Source: three-view drawing plus pictorial views. Frame: mm from the lowest corner of the part. Coordinates: 2 decimals unless noted, no trailing zeros. Loops run counter-clockwise (first coordinate to the right, second up) from the corner with the lowest first, then second, coordinate; pieces in that order, holes last. Notation, with made-up numbers: M -26,-40 L 9,-40 A4 ccw 9,-36 Z; hole C -18,-24 d10. An arc over 180 degrees is marked long. Use a Markdown table: item, result. Add a question column.
1. Section B-B on z = 5. Output: boundary loops of the cut face in (x, y).
2. Section D-D on x = 18. Output: boundary loops of the cut face in (y, z), then the cut area to 3 significant figures.
3. Pin query (flat end, axial travel): pin 1 (6 mm diameter, centred on x = 38, y = 9, fed in from +Z); pin 2 (2 mm diameter, centred on y = 3, z = 3.5, fed in from +X); pin 3 (2 mm diameter, centred on y = 20.5, z = 1, fed in from -X); pin 4 (4 mm diameter, centred on x = 79.5, z = 2.5, fed in from -Y). Return the tip coordinate at first contact, or that it passes through.
4. Line query: L1, parallel to Y at x = 12.25, z = 5; L2, parallel to Y at x = 4.5, z = 5; L3, parallel to X at y = 7, z = 9.5. Output: solid intervals per line, ascending. Write a range as [from, to].
5. Section C-C on y = 13. Output: boundary loops of the cut face in (x, z), then the cut area to 3 significant figures.
6. Section A-A on x = 5. Output: boundary loops of the cut face in (y, z).
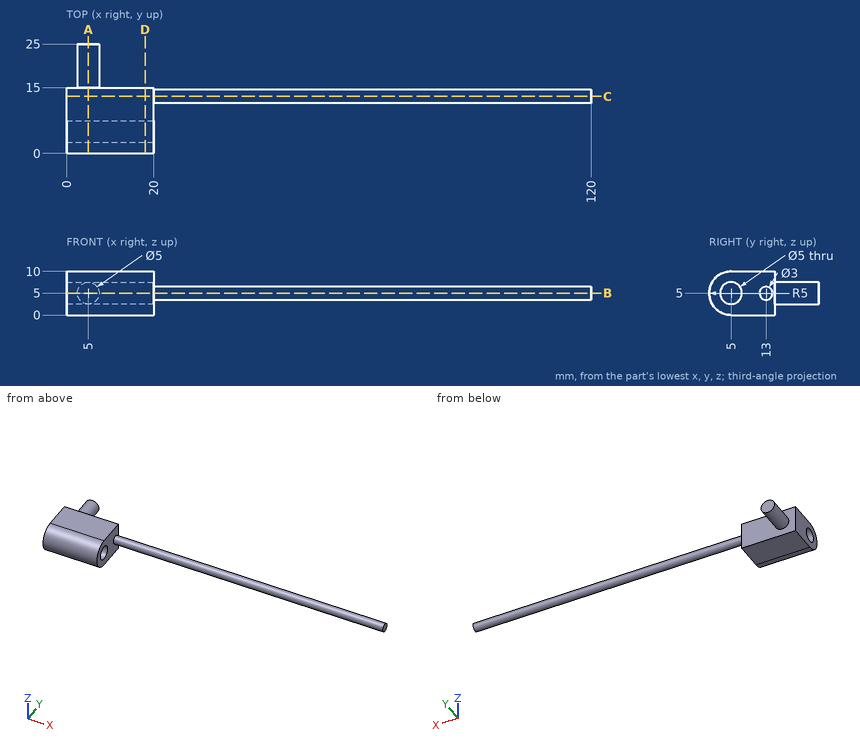
Answers below:
| question | item | result |
|---|---|---|
| 1 | outline | M 0,0 L 20,0 L 20,2.5 L 0,2.5 Z; M 0,7.5 L 20,7.5 L 20,11.5 L 120,11.5 L 120,14.5 L 20,14.5 L 20,15 L 7.5,15 L 7.5,25 L 2.5,25 L 2.5,15 L 0,15 Z |
| 2 | outline | M 5,0 L 15,0 L 15,10 L 5,10 A5 ccw Z; hole C 5,5 d5 |
| 2 | area | 120 mm² |
| 3 | pin 1 | stops at z = 6.12 |
| 3 | pin 2 | stops at x = 20 |
| 3 | pin 3 | passes through |
| 3 | pin 4 | stops at y = 11.59 |
| 4 | L1 | y = [0, 2.5], [7.5, 15] |
| 4 | L2 | y = [0, 2.5], [7.5, 25] |
| 4 | L3 | x = [0, 20] |
| 5 | outline | M 0,0 L 20,0 L 20,3.5 L 120,3.5 L 120,6.5 L 20,6.5 L 20,10 L 0,10 Z |
| 5 | area | 500 mm² |
| 6 | outline | M 5,0 L 15,0 L 15,2.5 L 25,2.5 L 25,7.5 L 15,7.5 L 15,10 L 5,10 A5 ccw Z; hole C 5,5 d5 |
